Part print with two shaded views. Sizes in mm from the minimum x, y, z corner. Round coordinates to 2 decimals unless told otherwise and drop trailing zeros. Loops run counter-clockwise (first coordinate to the right, second up) from the corner with the lowest first, then second, coordinate; pieces in that order, holes last. Notation, with made-up numbers: (-37.75, 32.5) -> (-9.75, 32.5) arc R32 cw to (-9.75, 70.5) -> close; hole circle Ø5 at (64, -25). An arc over 180 degrees is marked (long way). Use a Markdown table: item, result. Add a question column.
Item 1: Cut at A-A, the plane y = 179.5. List the corners of the cut face in (x, z).
Item 2: Cut at C-C, the plane y = 49.75. State how many separate pieces and enclosed holes the cut face has, plus the area to 4 significant figures.
Item 3: Two-plate mould, pull along Z, no slides. Class the marked faces 1 and 2: pulls with the +Z half, pulls with the -Z half, needs draft (parallel to the pull), parting line crosses it, or undercut.
Item 4: Probe line 1 (X direction, y = 179, z = 1.9); line 2 (X direction, y = 174.5, z = 1.45). List the from-to ranges inside material, lowest first. Write a range as [from, to].
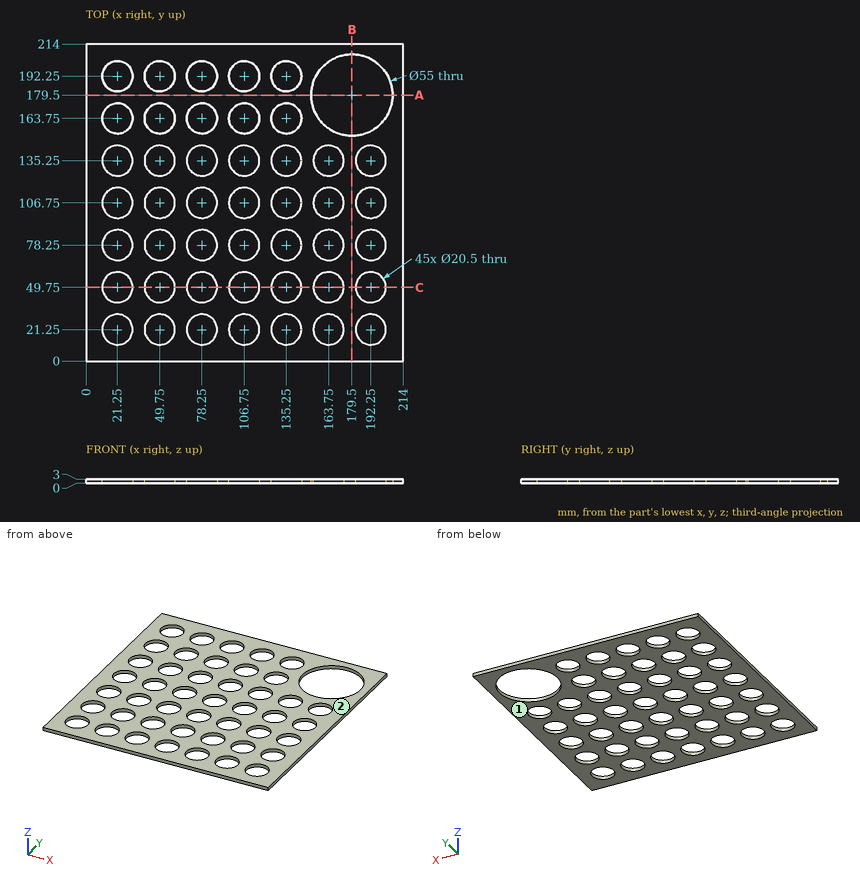
A:
| question | item | result |
|---|---|---|
| 1 | outline | (0, 0) -> (152, 0) -> (152, 3) -> (0, 3) -> close; (207, 0) -> (214, 0) -> (214, 3) -> (207, 3) -> close |
| 2 | separate pieces | 8 |
| 2 | enclosed holes | 0 |
| 2 | area | 211.5 mm^2 |
| 3 | face 1 | pulls with the -Z half |
| 3 | face 2 | pulls with the +Z half |
| 4 | line 1 | x = [0, 152], [207, 214] |
| 4 | line 2 | x = [0, 152.46], [206.54, 214] |
